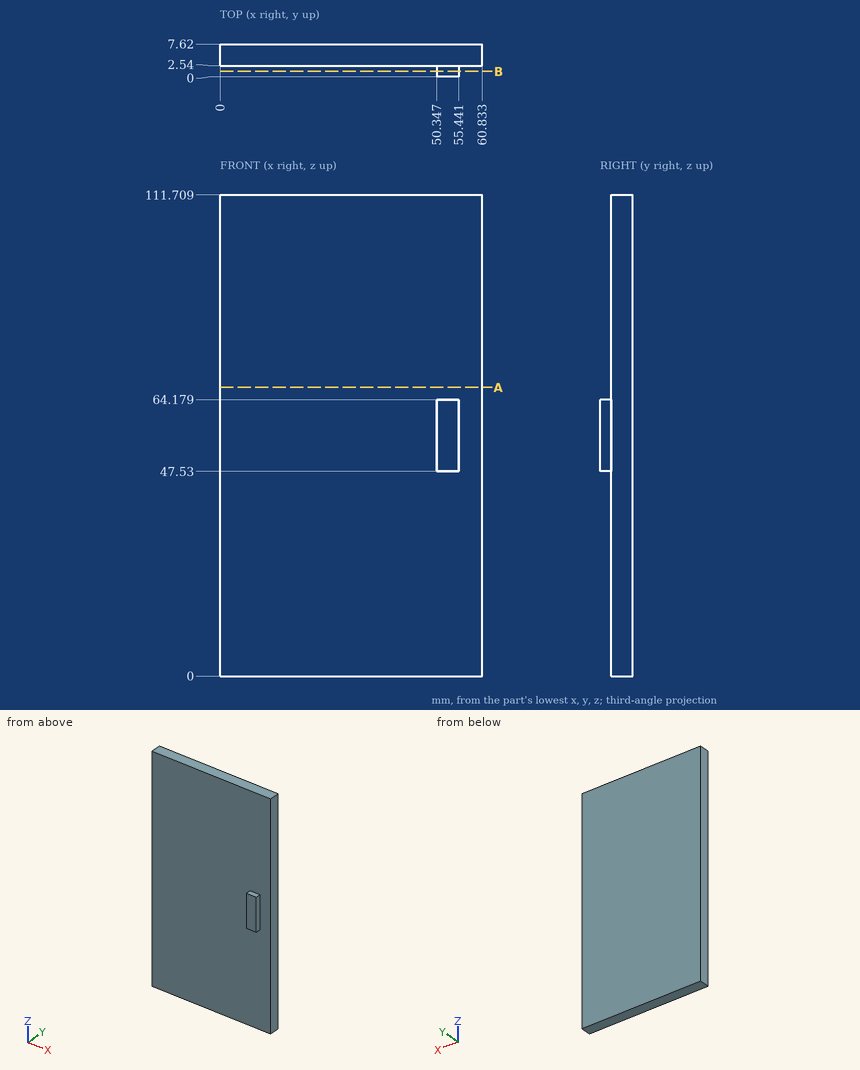
Answer from the drawing. Dimensions are ordinates in mm from the lowest x, y and z of the part. Give positions to 0.01 mm unless a question says otherwise; leave off trailing zeros. Loops run counter-clockwise (first coordinate to the right, second up) from the corner with the lowest first, then second, coordinate; pieces in that order, holes last.
Item 1: Each of these flat-tipped pins is pushed along its axis until it touches: pin 1 Ø2 at (x, z) = (25.5, 55.5) entering from -Y; pin 2 Ø0.8 at (y, z) = (1, 55.5) entering from -X; pin 3 Ø1.3 at (x, y) = (51.5, 1) entering from -Z. Where does it stop, or does it pass through?
Derived:
pin 1: stops at y = 2.54
pin 2: stops at x = 50.35
pin 3: stops at z = 47.53
Item 2: A cutting plane is placed at B-B (y = 1.25). Give the vertices of the cut face in (x, z).
Derived:
outline: (50.35, 47.53) - (55.44, 47.53) - (55.44, 64.18) - (50.35, 64.18) - close
Item 3: A cutting plane is placed at A-A (z = 67). Give the vertices of the cut face in (x, y), then the cut area to 3 significant figures.
Derived:
outline: (0, 2.54) - (60.83, 2.54) - (60.83, 7.62) - (0, 7.62) - close
area: 309 mm2
Item 4: Find the intervals of material crossed by line 1 along Y through (x, z) = (21, 73); line 2 along X through (y, z) = (2, 56.5), in increasing order.
Derived:
line 1: y = 2.54 to 7.62
line 2: x = 50.35 to 55.44
